```python
from build123d import *

# Parameters (mm, degrees)
SKETCH1_R               = 60
BOSS_EXTRUDE1_DEPTH     = 5
SKETCH2_W               = 10
SKETCH2_H               = 34
CUT_EXTRUDE1_DEPTH      = 1
CUT_EXTRUDE1_DEPTH_BACK = 6
SKETCH3_W               = 24
SKETCH3_H               = 10
BOSS_EXTRUDE2_DEPTH     = 10
SKETCH4_W               = 42
SKETCH4_H               = 33
CUT_EXTRUDE2_DEPTH      = 2
BOSS_EXTRUDE3_DEPTH     = 15
SKETCH6_R               = 2
CUT_EXTRUDE3_DEPTH      = 10


with BuildPart() as part:
    # Sketch1 → Boss-Extrude1 (new body)
    with BuildSketch(Plane(origin=(0, 0, 0), x_dir=(1, 0, 0), z_dir=(0, 1, 0))):
        Circle(SKETCH1_R)
    extrude(amount=BOSS_EXTRUDE1_DEPTH)

    # Sketch2 → Cut-Extrude1 (cut, two sides)
    with BuildSketch(Plane(origin=(0, 5, 0), x_dir=(1, 0, 0), z_dir=(0, 1, 0))) as cut_extrude1_sk:
        with Locations((-50, 0)):
            Rectangle(SKETCH2_W, SKETCH2_H)
        with Locations((50, 0)):
            Rectangle(SKETCH2_W, SKETCH2_H)
    extrude(amount=CUT_EXTRUDE1_DEPTH, mode=Mode.SUBTRACT)
    extrude(cut_extrude1_sk.sketch, amount=-CUT_EXTRUDE1_DEPTH_BACK, mode=Mode.SUBTRACT)

    # Sketch3 → Boss-Extrude2 (add)
    with BuildSketch(Plane(origin=(0, 5, 0), x_dir=(1, 0, 0), z_dir=(0, 1, 0))):
        with Locations((-33, -11.5)):
            Rectangle(SKETCH3_W, SKETCH3_H)
        with Locations((-33, 11.5)):
            Rectangle(SKETCH3_W, SKETCH3_H)
        with Locations((33, -11.5)):
            Rectangle(SKETCH3_W, SKETCH3_H)
        with Locations((33, 11.5)):
            Rectangle(SKETCH3_W, SKETCH3_H)
    extrude(amount=BOSS_EXTRUDE2_DEPTH)

    # Sketch4 → Cut-Extrude2 (cut)
    with BuildSketch(Plane(origin=(0, 5, 0), x_dir=(1, 0, 0), z_dir=(0, 1, 0))):
        Rectangle(SKETCH4_W, SKETCH4_H)
    extrude(amount=-CUT_EXTRUDE2_DEPTH, mode=Mode.SUBTRACT)

    # Sketch5 → Boss-Extrude3 (add)
    with BuildSketch(Plane(origin=(0, 5, 0), x_dir=(1, 0, 0), z_dir=(0, 1, 0))):
        with BuildLine():
            Line((-56.742840958, 19.5), (56.742840958, 19.5))
            ThreePointArc((56.742840958, 19.5), (0, 60), (-56.742840958, 19.5))
        make_face()
        with BuildLine():
            Line((-56.742840958, -19.5), (56.742840958, -19.5))
            ThreePointArc((56.742840958, -19.5), (0, -60), (-56.742840958, -19.5))
        make_face()
    extrude(amount=BOSS_EXTRUDE3_DEPTH)

    # Sketch6 → Cut-Extrude3 (cut)
    with BuildSketch(Plane(origin=(0, 20, 0), x_dir=(1, 0, 0), z_dir=(0, 1, 0))):
        with Locations((30, -40)):
            Circle(SKETCH6_R)
        with Locations((-30, -40)):
            Circle(SKETCH6_R)
        with Locations((30, 40)):
            Circle(SKETCH6_R)
        with Locations((-30, 40)):
            Circle(SKETCH6_R)
    extrude(amount=-CUT_EXTRUDE3_DEPTH, mode=Mode.SUBTRACT)

    # Sketch7 → Revolve1 (revolve)
    with BuildSketch(Plane(origin=(0, 0, 0), x_dir=(0, 0, -1), z_dir=(1, 0, 0))):
        with BuildLine():
            Line((-39.75, 0), (-39.75, -6.5))
            ThreePointArc((-39.75, -6.5), (-29.119335131, -4.825340555), (-19.5, 0))
            Line((-19.5, 0), (-39.75, 0))
        make_face()
    revolve(axis=Axis((0, 0, 39.75), (0, -1, 0)))


solid = part.part
```
The listing builds one solid part. Answer for the finished solid, in the listing's coordinates (mm). A direction names the side the tool comes from. Coordinates: 2 decimals unless noted, no trailing zeros. Write each loop counter-clockwise with the first axis right and the second up, starting at its lowest first coordinate (ties: lowest second). Pieces come first, ordered by that corner, then holes. Notation, with made-up numbers: (-5, 33) -> (12, 33) arc R20 cw to (12, 58) -> close; hole circle Ø3 at (70.25, 11.25). An arc over 180 degrees is marked (long way). Write each question's results on one line, items separated by ' | '. Start each with the question number.
1) A tool of negligible diameter and unlimited length cuts with its end or side. For faces 1 (the flat face through (-33, 5, 0)), 2 (the flat face through (-30, 10, -40)), 3 (the flat face through (50, 3, -17)), from which of +Z, -Z, +X, -X, +Y, -Y can it reach the whole face along a straight path? Write none if from no direction.
2) A cutting plane is placed at D-D (x = 30). Determine the outline of the cut face in (y, z).
3) Flat-ended cylindrical pins translate along their axes: pin 1 Ø1.5 at (y, z) = (2.5, -2) entering from +X; pin 2 Ø4.5 at (x, y) = (13.5, 15.5) entering from -Z; pin 3 Ø10 at (y, z) = (-1.5, 35.5) entering from -X. Find the tip coordinate at first contact, or state that the pin passes through.
4) Straight lines are drawn through the part: probe 1 along X at (y, z) = (1, 13.5); probe 2 along Z at (x, y) = (41, 7.75); probe 3 along Z at (x, y) = (-30, 13). For each, find the intervals that lie inside material, in ascending order.
5) A cutting plane is placed at C-C (x = -52.5). Determine the outline of the cut face in (y, z), then the cut area to 3 significant figures.
6) A cutting plane is placed at B-B (y = 7.75). Determine the outline of the cut face in (x, z), then the cut area to 3 significant figures.
7) For a pull along X with two mould halves and no side action, classify faces 4 (the cylindrical face through (30.923, 15.07, -38.226)), 5 (the flat face through (33, 10, 16.5)) as +X half, -X half, draft (parallel to the pull), parting line (faces both ways), or undercut.
8) A cutting plane is placed at A-A (z = 0). Determine the outline of the cut face in (x, y).
Values follow:
1) face 1: +X, -X, +Y | face 2: +Y | face 3: +Y, -Y
2) outline: (0, -51.96) -> (20, -51.96) -> (20, -42) -> (10, -42) -> (10, -38) -> (20, -38) -> (20, -19.5) -> (5, -19.5) -> (5, -16.5) -> (15, -16.5) -> (15, -6.5) -> (5, -6.5) -> (5, 6.5) -> (15, 6.5) -> (15, 16.5) -> (5, 16.5) -> (5, 19.5) -> (20, 19.5) -> (20, 38) -> (10, 38) -> (10, 42) -> (20, 42) -> (20, 51.96) -> (0, 51.96) -> close
3) pin 1: x = 59.99 | pin 2: z = -58.94 | pin 3: x = -51.53
4) probe 1: -58.46 to -55, -45 to 45, 55 to 58.46 | probe 2: -43.81 to -19.5, -16.5 to -6.5, 6.5 to 16.5, 19.5 to 43.81 | probe 3: -51.96 to -42, -38 to -19.5, -16.5 to -6.5, 6.5 to 16.5, 19.5 to 38, 42 to 51.96
5) outline: (0, -29.05) -> (20, -29.05) -> (20, -19.5) -> (5, -19.5) -> (5, -17) -> (0, -17) -> close; (0, 17) -> (5, 17) -> (5, 19.5) -> (20, 19.5) -> (20, 29.05) -> (0, 29.05) -> close | area: 407 mm²
6) outline: (-56.74, -19.5) arc R60 ccw to (56.74, -19.5) -> close; (-56.74, 19.5) -> (56.74, 19.5) arc R60 ccw to start; (-45, -16.5) -> (-21, -16.5) -> (-21, -6.5) -> (-45, -6.5) -> close; (-45, 6.5) -> (-21, 6.5) -> (-21, 16.5) -> (-45, 16.5) -> close; (21, -16.5) -> (45, -16.5) -> (45, -6.5) -> (21, -6.5) -> close; (21, 6.5) -> (45, 6.5) -> (45, 16.5) -> (21, 16.5) -> close | area: 7,670 mm²
7) face 4: undercut | face 5: draft
8) outline: (-60, 0) -> (-55, 0) -> (-55, 5) -> (-60, 5) -> close; (-45, 0) -> (45, 0) -> (45, 5) -> (21, 5) -> (21, 3) -> (-21, 3) -> (-21, 5) -> (-45, 5) -> close; (55, 0) -> (60, 0) -> (60, 5) -> (55, 5) -> close
